Geometry check sheet. Reference: the model listing, model coordinates, mm. A direction names the side the tool comes from. Coordinates: 2 decimals unless noted, no trailing zeros. Write each loop counter-clockwise with the first axis right and the second up, starting at its lowest first coordinate (ties: lowest second). Pieces come first, ordered by that corner, then holes. Notation, with made-up numbers: (39, 73) -> (65, 73) arc R28 cw to (65, 110) -> close; hole circle Ø6 at (22.5, -25.75). An arc over 180 degrees is marked (long way). Answer in a Markdown table with one row per item. Add a question column.
1. Depth check by flat-ended pin: P1, Ø1.5, axis at x = -11.5, z = 1.5, coming from the -Y side; P2, Ø1.5, axis at y = 8.5, z = 3, coming from the -X side; P3, Ø2.5, axis at y = 4, z = 1.5, coming from the -X side. Enter the tip coordinate at first touch or a pass-through.
2. Scan lines: L1, parallel to X at y = 10, z = 4.75; L2, parallel to Y at x = 0, z = 1.95; L3, parallel to Y at x = 10.8, z = 5.05. Record each from-to range of solid material in increasing order. Write a range as from..to.
3. Cross-section at B-B on x = 0. Record the cut outline in (y, z).
4. Cross-section at C-C on y = 9.5. Record the cut outline in (x, z), and give its area (3 significant figures).
5. Mould release check, pull along Y, two halves, no side actions. Record for faces 1 (the cylindrical face through (-9.32, 9.39, 5.46)), 2 (the flat face through (5, 3, 1)), 3 (the flat face through (11, 13, 1)), 4 (the flat face through (0, 14, 4)): pulls with the +Y half, pulls with the -Y half, needs draft (parallel to the pull), parting line crosses it, or undercut.
6. Cross-section at D-D on z = 6.75. Record the cut outline in (x, y), and give its area (3 significant figures).
7. Set-up check for faces 5 (the flat face through (0, 3, 3)), 6 (the cylindrical face through (0, -5, 1)), 7 (the flat face through (-8.2, 11.5, 1.5)): record each of +Z, -Z, +X, -X, +Y, -Y from which the full face is reachable in a straight line by a thin tool's end or side.
8. Cross-section at A-A on y = 1. Record the cut outline in (x, z), and give its area (3 significant figures).
```python
from build123d import *

# Parameters (mm, degrees)
F0_R     = 2.6
F0_R_2   = 1.6
F1_DEPTH = 3
F2_R     = 1.6
F3_DEPTH = 5
F5_DEPTH = 3


with BuildPart() as f1:
    # F0 (on Top) → F1 (new body)
    with BuildSketch(Plane.XY):
        with BuildLine():
            Line((-5, 6), (-5, 0))
            ThreePointArc((-5, 0), (0, -5), (5, 0))
            Line((5, 0), (5, 6))
            Line((5, 6), (10.8, 6))
            ThreePointArc((10.8, 6), (14.8, 10), (10.8, 14))
            Line((10.8, 14), (0, 14))
            Line((0, 14), (-10.8, 14))
            ThreePointArc((-10.8, 14), (-14.8, 10), (-10.8, 6))
            Line((-10.8, 6), (-5, 6))
        make_face()
        Circle(F0_R, mode=Mode.SUBTRACT)
        with Locations((-10.8, 10)):
            Circle(F0_R_2, mode=Mode.SUBTRACT)
        with Locations((10.8, 10)):
            Circle(F0_R_2, mode=Mode.SUBTRACT)
    extrude(amount=F1_DEPTH)

    # F2 (on face) → F3 (join)
    with BuildSketch(Plane.XY.offset(3)):
        with BuildLine():
            ThreePointArc((10.8, 6), (14.8, 10), (10.8, 14))
            Line((10.8, 14), (-10.8, 14))
            ThreePointArc((-10.8, 14), (-14.8, 10), (-10.8, 6))
            Line((-10.8, 6), (-5, 6))
            Line((-5, 6), (5, 6))
            Line((5, 6), (10.8, 6))
        make_face()
        with Locations((-10.8, 10)):
            Circle(F2_R, mode=Mode.SUBTRACT)
        with Locations((10.8, 10)):
            Circle(F2_R, mode=Mode.SUBTRACT)
    extrude(amount=F3_DEPTH)

    # F4 (on face) → F5 (cut)
    with BuildSketch(Plane(origin=(0, 0, 0), x_dir=(1, 0, 0), z_dir=(0, 0, -1))):
        Polygon((9.067949, -13), (12.532051, -13), (14.264102, -10), (12.532051, -7), (9.067949, -7), (7.335898, -10), align=None)
        Polygon((-12.532051, -13), (-9.067949, -13), (-7.335898, -10), (-9.067949, -7), (-12.532051, -7), (-14.264102, -10), align=None)
    extrude(amount=-F5_DEPTH, mode=Mode.SUBTRACT)


solid = f1.part
```
Results found:
| question | item | result |
|---|---|---|
| 1 | P1 | stops at y = 6 |
| 1 | P2 | stops at x = -14.73 |
| 1 | P3 | stops at x = -5 |
| 2 | L1 | x = -14.8..-12.4, -9.2..9.2, 12.4..14.8 |
| 2 | L2 | y = -5..-2.6, 2.6..14 |
| 2 | L3 | y = 6..8.4, 11.6..14 |
| 3 | outline | (-5, 0) -> (-2.6, 0) -> (-2.6, 3) -> (-5, 3) -> close; (2.6, 0) -> (14, 0) -> (14, 8) -> (6, 8) -> (6, 3) -> (2.6, 3) -> close |
| 4 | outline | (-14.77, 0) -> (-13.98, 0) -> (-13.98, 3) -> (-12.32, 3) -> (-12.32, 8) -> (-14.77, 8) -> close; (-9.28, 3) -> (-7.62, 3) -> (-7.62, 0) -> (7.62, 0) -> (7.62, 3) -> (9.28, 3) -> (9.28, 8) -> (-9.28, 8) -> close; (12.32, 3) -> (13.98, 3) -> (13.98, 0) -> (14.77, 0) -> (14.77, 8) -> (12.32, 8) -> close |
| 4 | area | 168 mm^2 |
| 5 | face 1 | undercut |
| 5 | face 2 | needs draft |
| 5 | face 3 | undercut |
| 5 | face 4 | pulls with the +Y half |
| 6 | outline | (-10.8, 6) -> (10.8, 6) arc R4 ccw to (10.8, 14) -> (-10.8, 14) arc R4 ccw to start; hole circle Ø3.2 at (-10.8, 10); hole circle Ø3.2 at (10.8, 10) |
| 6 | area | 207 mm^2 |
| 7 | face 5 | +Z, +X, -X, -Y |
| 7 | face 6 | +Z, -Z, -Y |
| 7 | face 7 | -Z |
| 8 | outline | (-5, 0) -> (-2.4, 0) -> (-2.4, 3) -> (-5, 3) -> close; (2.4, 0) -> (5, 0) -> (5, 3) -> (2.4, 3) -> close |
| 8 | area | 15.6 mm^2 |
